Read the model definition and answer for the solid it produces. Units are mm, in the model's axes. Coordinates: 2 decimals unless noted, no trailing zeros. Write each loop counter-clockwise with the first axis right and the second up, starting at its lowest first coordinate (ties: lowest second). Pieces come first, ordered by that corner, then holes. Notation, with made-up numbers: (6, 6.5) -> (32, 6.5) arc R35 ccw to (32, 42.5) -> close; hole circle Ø4 at (43, 19.25). An arc over 180 degrees is marked (long way). Answer in a Markdown table with one row per item. Add a question column.
Item 1: Section A-A on z = 0 is taken. Write down the section's boundary in (x, y), then the cut area to 3 significant figures.
Item 2: Straight lines are drawn through the part: line 1 (Z direction, x = 90, y = 3); line 2 (Z direction, x = 116.8, y = 1.8); line 3 (X direction, y = 2.8, z = 5). For each, find the intervals that lie inside material, in ascending order. Write a range as from..to.
Item 3: Section C-C on x = 75 is taken. Write down the section's boundary in (y, z), then the cut area to 3 significant figures.
Item 4: Section B-B on y = 2.4 is taken. Count the separate pieces of the cut face and the enclosed holes in it, then the cut area to 3 significant figures.
```python
from build123d import *

# Parameters (mm, degrees)
SALIENTE_EXTRUIR1_DEPTH = 4
CROQUIS2_R              = 84.42
CROQUIS2_R_2            = 2
CORTAR_EXTRUIR1_DEPTH   = 4
CROQUIS3_R              = 2
CORTAR_EXTRUIR2_DEPTH   = 10


with BuildPart() as part:
    # Croquis1 → Saliente-Extruir1 (new body)
    with BuildSketch(Plane(origin=(0, 0, 0), x_dir=(1, 0, 0), z_dir=(0, 1, 0))):
        with BuildLine():
            Line((-125, -123.5), (125, -123.5))
            Line((125, -123.5), (125, 113.5))
            ThreePointArc((125, 113.5), (122.071067812, 120.571067812), (115, 123.5))
            Line((115, 123.5), (-115, 123.5))
            ThreePointArc((-115, 123.5), (-122.071067812, 120.571067812), (-125, 113.5))
            Line((-125, 113.5), (-125, -123.5))
        make_face()
    extrude(amount=SALIENTE_EXTRUIR1_DEPTH)

    # Croquis2 → Cortar-Extruir1 (cut)
    with BuildSketch(Plane(origin=(0, 4, 0), x_dir=(1, 0, 0), z_dir=(0, 1, 0))):
        with Locations(Location((0, 0, 0), (0, 0, 270))):
            Circle(CROQUIS2_R)
        with Locations(Location((-90, 5, 0), (0, 0, 270))):
            Circle(CROQUIS2_R_2)
        with Locations(Location((-90, -5, 0), (0, 0, 270))):
            Circle(CROQUIS2_R_2)
        with Locations(Location((90, -5, 0), (0, 0, 90))):
            Circle(CROQUIS2_R_2)
        with Locations(Location((90, 5, 0), (0, 0, 90))):
            Circle(CROQUIS2_R_2)
    extrude(amount=-CORTAR_EXTRUIR1_DEPTH, mode=Mode.SUBTRACT)

    # Croquis3 → Cortar-Extruir2 (cut)
    with BuildSketch(Plane(origin=(0, 4, 0), x_dir=(1, 0, 0), z_dir=(0, 1, 0))):
        with Locations(Location((-116.8, 85.7, 0), (0, 0, 270))):
            Circle(CROQUIS3_R)
        with Locations(Location((-116.8, 55.65, 0), (0, 0, 270))):
            Circle(CROQUIS3_R)
        with Locations(Location((-116.8, -10.55, 0), (0, 0, 270))):
            Circle(CROQUIS3_R)
        with Locations(Location((-116.8, -40.6, 0), (0, 0, 270))):
            Circle(CROQUIS3_R)
        with Locations(Location((116.8, -40.6, 0), (0, 0, 90))):
            Circle(CROQUIS3_R)
        with Locations(Location((116.8, -10.55, 0), (0, 0, 90))):
            Circle(CROQUIS3_R)
        with Locations(Location((116.8, 55.65, 0), (0, 0, 90))):
            Circle(CROQUIS3_R)
        with Locations(Location((116.8, 85.7, 0), (0, 0, 90))):
            Circle(CROQUIS3_R)
    extrude(amount=-CORTAR_EXTRUIR2_DEPTH, mode=Mode.SUBTRACT)


solid = part.part
```
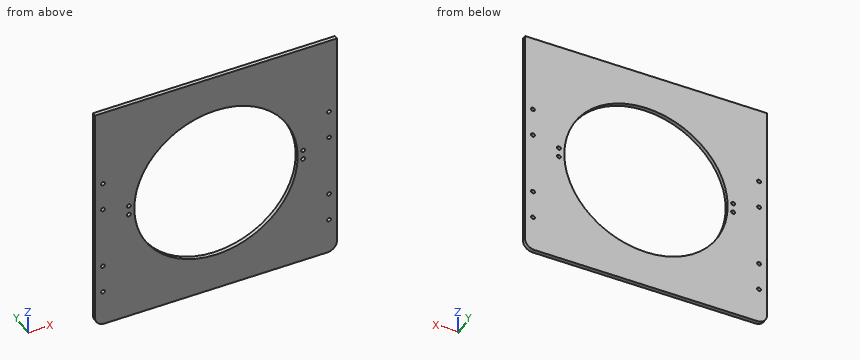
Results below:
| question | item | result |
|---|---|---|
| 1 | outline | (-125, 0) -> (-84.42, 0) -> (-84.42, 4) -> (-125, 4) -> close; (84.42, 0) -> (125, 0) -> (125, 4) -> (84.42, 4) -> close |
| 1 | area | 325 mm2 |
| 2 | line 1 | z = -123.5..-7, -3..3, 7..123.5 |
| 2 | line 2 | z = -123.34..-87.7, -83.7..-57.65, -53.65..8.55, 12.55..38.6, 42.6..123.5 |
| 2 | line 3 | x = -125..-92, -88..-84.27, 84.27..88, 92..125 |
| 3 | outline | (0, -123.5) -> (4, -123.5) -> (4, -38.75) -> (0, -38.75) -> close; (0, 38.75) -> (4, 38.75) -> (4, 123.5) -> (0, 123.5) -> close |
| 3 | area | 678 mm2 |
| 4 | separate pieces | 1 |
| 4 | enclosed holes | 13 |
| 4 | area | 39,200 mm2 |
